Model file for the job. Use its own axes, mm. A direction names the side the tool comes from. Round coordinates to 2 decimals unless told otherwise and drop trailing zeros. Loops run counter-clockwise (first coordinate to the right, second up) from the corner with the lowest first, then second, coordinate; pieces in that order, holes last. Notation, with made-up numbers: (-37, -20.75) - (20, -20.75) arc R27 cw to (20, 11.25) - close; hole circle Ø8 at (45, 40.5). An arc over 180 degrees is marked (long way). Use one line per item in the form item = value.
Autodesk Inventor part; units mm, degrees
ref_plane "YZ Plane" through (0, 0, 0) normal (1, 0, 0) x (0, 1, 0)
ref_plane "XZ Plane" through (0, 0, 0) normal (0, 1, 0) x (-1, 0, 0)
ref_plane "XY Plane" through (0, 0, 0) normal (0, 0, 1) x (1, 0, 0)
sketch "Sketch1" plane through (0, 0, 0) normal (0, 1, 0) x (-1, 0, 0)
  arc A0 (5.4, 2.6153) -> (5.4, -2.6153) centre (0, 0) ccw
  line L0 (3.75, 3.75) -> (-3.75, 3.75)
  line L1 (-3.75, 3.75) -> (-3.75, -3.75)
  line L2 (-3.75, -3.75) -> (3.75, -3.75)
  line L3 (3.75, -3.75) -> (3.75, 3.75)
  line L4 (3.75, 3.75) -> (-3.75, -3.75) construction
  line L5 (-3.75, 3.75) -> (3.75, -3.75) construction
  line L6 (5.4, -2.6153) -> (5.4, 2.6153)
  circle A1 centre (2.5, 2.5) radius 1.1
  circle A2 centre (2.5, -2.5) radius 1.1
  circle A3 centre (-2.5, 2.5) radius 1.1
  circle A4 centre (-2.5, -2.5) radius 1.1
  point P0 (-6, 0)
  dimension "d0" = 12
  dimension "d1" = 7.5
  dimension "d2" = 7.5
  dimension "d3" = 11.4
  dimension "d4" = 2.2
  dimension "d7" = 5
  dimension "d10" = 5
extrude "Extrusion1" add sketch "Sketch1" along normal blind 5.8 contours L6 A0
extrude "Extrusion2" add sketch "Sketch1" along normal blind 9.8 contours L3 L2 L1 L0 | A1 | A2 | A3 | A4
extrude "Extrusion3" add sketch "Sketch1" against normal blind 5 contours A1 | A2 | A3 | A4
fillet "Fillet1" radius 0.2 4 edges at (0, 9.8, -3.75) (-3.75, 9.8, 0) (0, 9.8, 3.75) (3.75, 9.8, 0)
properties part number "D6C90 F1 LFS"
1. Tool access for faces 1 (the flat face through (3.75, 8, 0)), 2 (the flat face through (0, 8, 3.75)), 3 (the cylindrical face through (-3.55, -2.46, -2.17)), 4 (the flat face through (-3.75, 8, 0)): list every direction of +Z, -Z, +X, -X, +Y, -Y with a clear straight run to the whole face (end or side of a thin tool).
Geometry check:
face_1 = +Z, -Z, +X, +Y
face_2 = +Z, +X, -X, +Y
face_3 = -Y
face_4 = +Z, -Z, -X, +Y
2. Cut at A-A, the plane x = 0. Give the cut face in (y, z), plus the area to 3 significant figures.
Geometry check:
outline = (0, -6) - (5.8, -6) - (5.8, -3.75) - (9.6, -3.75) arc R0.2 ccw to (9.8, -3.55) - (9.8, 3.55) arc R0.2 ccw to (9.6, 3.75) - (5.8, 3.75) - (5.8, 6) - (0, 6) - close
area = 99.6 mm^2
3. Wall check: probe 1 along Y at (x, z) = (-1.5, -0.5); probe 2 along Y at (x, z) = (4, -2); probe 3 along Z at (x, y) = (-3, 9.25). Give the ranges that are in metal, low to high.
Geometry check:
probe_1 = 0 to 9.8
probe_2 = 0 to 5.8
probe_3 = -3.75 to 3.75
4. Pull direction Z, two halves, no side cores. Call faces 5 (the cylindrical face through (1.45, -2.46, 2.83)), 6 (the flat face through (0, 8, -3.75)), 7 (the cylindrical face through (6, 3, 0)): +Z half, -Z half, draft (parallel to the pull), parting line (faces both ways), or undercut.
Geometry check:
face_5 = undercut
face_6 = -Z half
face_7 = parting line
5. Flat gauge pins, fed straight in: pin 1 (4 mm diameter, centred on x = 0, y = 8, fed in from +Z); pin 2 (4 mm diameter, centred on y = 5, z = -4, fed in from -X); pin 3 (1.1 mm diameter, centred on y = 8, z = 1, fed in from -X); pin 4 (3 mm diameter, centred on x = -1.5, y = 7.5, fed in from -Z). Where does each tip first touch, or does it go through?
Geometry check:
pin_1 = 3.75
pin_2 = -5.4
pin_3 = -3.75
pin_4 = -3.75
6. Cut at B-B, the plane y = -3.75. Give the cut face in (x, z), plus the area to 3 significant figures.
Geometry check:
outline = circle Ø2.2 at (-2.5, -2.5); circle Ø2.2 at (-2.5, 2.5); circle Ø2.2 at (2.5, -2.5); circle Ø2.2 at (2.5, 2.5)
area = 15.2 mm^2
7. Cut at D-D, the plane y = 8.5. Give the cut face in (x, z), plus the area to 4 significant figures.
Geometry check:
outline = (-3.75, -3.75) - (3.75, -3.75) - (3.75, 3.75) - (-3.75, 3.75) - close
area = 56.25 mm^2
8. Cut at C-C, the plane z = 0. Give the cut face in (x, y).
Geometry check:
outline = (-5.4, 0) - (6, 0) - (6, 5.8) - (3.75, 5.8) - (3.75, 9.6) arc R0.2 ccw to (3.55, 9.8) - (-3.55, 9.8) arc R0.2 ccw to (-3.75, 9.6) - (-3.75, 5.8) - (-5.4, 5.8) - close
